Here's how the part is built. I have some questions about the finished solid (model axes, mm). A direction names the side the tool comes from. Round coordinates to 2 decimals unless told otherwise and drop trailing zeros. Write each loop counter-clockwise with the first axis right and the second up, starting at its lowest first coordinate (ties: lowest second). Pieces come first, ordered by that corner, then holes. Notation, with made-up numbers: (75.5, -14.75) - (87.5, -14.75) arc R19 cw to (87.5, 5.25) - close; hole circle Ø1 at (27, -3). An arc over 180 degrees is marked (long way). One line per question, with ' | ' between items. Start each with the question number.
(1) For faces 4 (the cylindrical face through (15.277, 42.064, 7.042)), 5 (the flat face through (78, 45, 12)), which set-ups out of +Z, -Z, +X, -X, +Y, -Y let a thin tool reach every point of the face, with its end or its side?
(2) Imagine slicing it at A-A (y = 38). Write out the boundary of the cut face in (x, z).
(3) Imagine slicing it at C-C (y = 68). Write out the boundary of the cut face in (x, z).
(4) Thinking about a two-plate mould opening in Y: for faces 1 (the flat face through (136.19, 19.77, 6.08)), 2 (the flat face through (9.361, 45, 5)), 3 (the cylindrical face through (135.88, 59.71, 6.08)), which applies, pulls with the +Y half, pulls with the -Y half, needs draft (parallel to the pull), parting line crosses it, or undercut?
(5) Imagine slicing it at B-B (z = 8). Write out the boundary of the cut face in (x, y), plus the area to 3 significant figures.
(6) Will this pin go through, and if not, where does the flat tip stop? pin 1 (3 mm diameter, centred on x = 134.36, y = 61.69, fed in from +Z).
(7) If I drill on L1, parallel to X at y = 44, z = 0.5; L2, parallel to X at y = 64, z = 0.75; L3, parallel to X at y = 46, z = 10.75, over which ranges is the centre line in solid material (lowest first)?
Solid Edge part; units mm, degrees
sketch "Sketch1" plane through (0, 0, 0) normal (0, 0, 1) x (1, 0, 0)
  line L0 (9.3609, 12.3736) -> (149.3609, 12.3736)
  line L1 (149.3609, 12.3736) -> (149.3609, 76.3736)
  line L2 (149.3609, 76.3736) -> (9.3609, 76.3736)
  line L3 (9.3609, 76.3736) -> (9.3609, 12.3736)
extrude "Protrusion1" add sketch "Sketch1" along normal blind 12
sketch "Sketch2" plane through (79.3609, 44.3736, 12) normal (0, 0, 1) x (1, 0, 0)
  line L0 (44.0192, 32) -> (70, 17)
  line L1 (70, 32) -> (70, 17)
  line L2 (44.0192, 32) -> (70, 32)
  line L3 (44.0192, -32) -> (70, -17)
  line L4 (70, -17) -> (70, -32)
  line L5 (70, -32) -> (44.0192, -32)
  dimension "D1" = 44.0192
extrude "ExtrudedCutout_2" cut sketch "Sketch2" against normal blind 12
sketch "Sketch3" plane through (79.3609, 44.3736, 12) normal (0, 0, 1) x (1, 0, 0)
  circle A0 centre (45, 0) radius 15
extrude "ExtrudedCutout_3" cut sketch "Sketch3" against normal blind 12
sketch "Sketch4" plane through (79.3609, 44.3736, 12) normal (0, 0, 1) x (0, 1, 0)
  circle A0 centre (0, -25) radius 2.5
  circle A1 centre (0, -65) radius 2.5
  circle A2 centre (17.3205, -35) radius 2.5
  circle A3 centre (-17.3205, -35) radius 2.5
  circle A4 centre (-17.3205, -55) radius 2.5
  circle A5 centre (17.3205, -55) radius 2.5
extrude "ExtrudedCutout_4" cut sketch "Sketch4" against normal blind 12
sketch "Sketch5" plane through (9.3609, 44.3736, 6) normal (-1, 0, 0) x (0, -1, 0)
  circle A0 centre (0, 2) radius 2.5
extrude "Cutout1" cut sketch "Sketch5" against normal blind 12
Check sheet entries:
1) face 4: -X | face 5: +Z, +X, -X, +Y, -Y
2) outline: (9.36, 0) - (110.78, 0) - (110.78, 12) - (9.36, 12) - close; (137.94, 0) - (149.36, 0) - (149.36, 12) - (137.94, 12) - close
3) outline: (9.36, 0) - (137.88, 0) - (137.88, 12) - (9.36, 12) - close
4) face 1: pulls with the -Y half | face 2: needs draft | face 3: undercut
5) outline: (9.36, 12.37) - (123.38, 12.37) - (149.36, 27.37) - (149.36, 61.37) - (123.38, 76.37) - (9.36, 76.37) - (9.36, 46.87) - (21.36, 46.87) - (21.36, 41.87) - (9.36, 41.87) - close; hole circle Ø5 at (104.36, 44.37); hole circle Ø30 at (124.36, 44.37); hole circle Ø5 at (114.36, 27.05); hole circle Ø5 at (114.36, 61.69); hole circle Ø5 at (134.36, 27.05); hole circle Ø5 at (134.36, 61.69); hole circle Ø5 at (144.36, 44.37) | area: 7,690 mm^2
6) pin 1: through
7) L1: 9.36 to 101.89, 106.83 to 109.37, 139.36 to 141.89, 146.83 to 149.36 | L2: 9.36 to 113.4, 115.33 to 133.4, 135.33 to 144.81 | L3: 9.36 to 102.46, 106.26 to 109.45, 139.27 to 142.46, 146.26 to 149.36
